Here's the drawing with two shaded views (mm, measured from the low corner). I have some questions. Coordinates: 2 decimals unless noted, no trailing zeros. Write each loop counter-clockwise with the first axis right and the second up, starting at its lowest first coordinate (ties: lowest second). Pieces come first, ordered by that corner, then holes.
Item 1: For P1, Ø5.5, axis at y = 6.5, z = 36.5, coming from the -X side; P2, Ø3.5, axis at y = 36.65, z = 36.65, coming from the -X side, each with a flat end and sliding along its axis, tell me the tip position at first contact or that it passes through.
Item 2: I want a section at C-C on y = 21.15. Please give me the cut outline in (x, z).
Item 3: I want a section at A-A on z = 36.65. Please give me the cut outline in (x, y).
Item 4: If I drill on probe 1 along Y at (x, z) = (6.3, 36.65); probe 2 along Y at (x, z) = (1.75, 36.65), over which ranges is the centre line in solid material (lowest first)?
Item 5: I want a section at B-B on x = 1.25. Please give me the cut outline in (y, z).
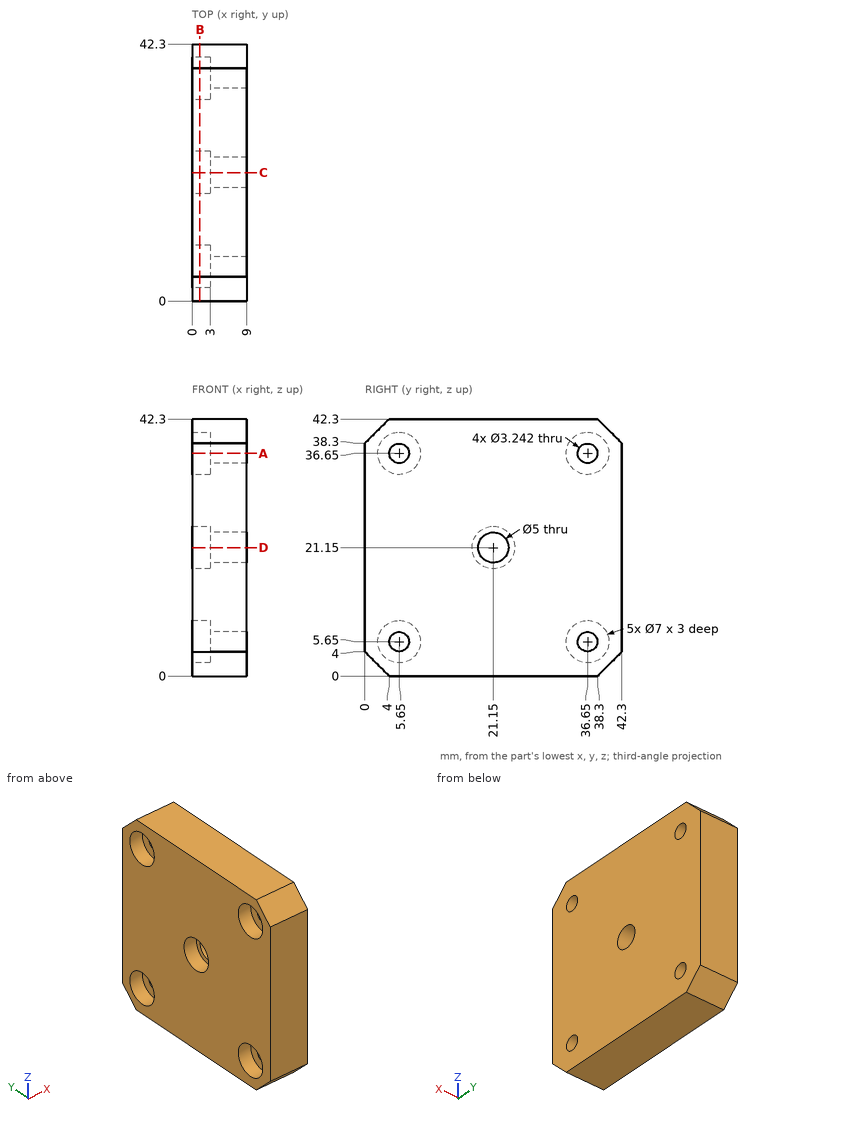
Response values:
1. P1: stops at x = 0
1. P2: stops at x = 3
2. outline: (0, 0) - (9, 0) - (9, 18.65) - (3, 18.65) - (3, 17.65) - (0, 17.65) - close; (0, 24.65) - (3, 24.65) - (3, 23.65) - (9, 23.65) - (9, 42.3) - (0, 42.3) - close
3. outline: (0, 0) - (9, 0) - (9, 4.03) - (3, 4.03) - (3, 2.15) - (0, 2.15) - close; (0, 9.15) - (3, 9.15) - (3, 7.27) - (9, 7.27) - (9, 35.03) - (3, 35.03) - (3, 33.15) - (0, 33.15) - close; (0, 40.15) - (3, 40.15) - (3, 38.27) - (9, 38.27) - (9, 42.3) - (0, 42.3) - close
4. probe 1: y = 0 to 4.03, 7.27 to 35.03, 38.27 to 42.3
4. probe 2: y = 0 to 2.15, 9.15 to 33.15, 40.15 to 42.3
5. outline: (0, 4) - (4, 0) - (38.3, 0) - (42.3, 4) - (42.3, 38.3) - (38.3, 42.3) - (4, 42.3) - (0, 38.3) - close; hole circle Ø7 at (5.65, 5.65); hole circle Ø7 at (5.65, 36.65); hole circle Ø7 at (21.15, 21.15); hole circle Ø7 at (36.65, 5.65); hole circle Ø7 at (36.65, 36.65)
